```python
from build123d import *

# Parameters (mm, degrees)
EXTRUDE_1_DEPTH     = 6.6
SKETCH_2_W          = 4
SKETCH_2_H          = 1.1
CUT_EXTRUDE_1_DEPTH = 6.6
EXTRUDE_2_DEPTH     = 1
SKETCH_4_W          = 3.4
SKETCH_4_H          = 0.4
EXTRUDE_3_DEPTH     = 3.9
CHAMFER_1_SIZE      = 0.1
CHAMFER_1_SIZE2     = 0.173205081
SKETCH_5_W          = 8
SKETCH_5_H          = 1.5
SKETCH_5_W_2        = 2
SKETCH_5_H_2        = 1.9
CUT_EXTRUDE_2_DEPTH = 1.4
SKETCH_6_W          = 0.25
SKETCH_6_H          = 0.8
SKETCH_6_H_2        = 0.9
EXTRUDE_5_DEPTH     = 2.6
SKETCH_7_W          = 0.25
SKETCH_7_H          = 0.4
EXTRUDE_6_DEPTH     = 1.4
SKETCH_8_W          = 0.3
SKETCH_8_H          = 0.2
EXTRUDE_7_DEPTH     = 1.4
SKETCH_9_W          = 0.3
SKETCH_9_H          = 3.7
EXTRUDE_8_DEPTH     = 0.01
SKETCH_10_W         = 2.6
SKETCH_10_H         = 1.6
EXTRUDE_9_DEPTH     = 0.25
FILLET_1_R          = 0.1


with BuildPart() as part:
    # 草图1 → 凸台-拉伸1 (new body)
    with BuildSketch(Plane.XY):
        with BuildLine():
            Line((-3.35, 1.15), (3.35, 1.15))
            ThreePointArc((3.35, 1.15), (3.597487373, 1.047487373), (3.7, 0.8))
            Line((3.7, 0.8), (3.7, 0.1))
            ThreePointArc((3.7, 0.1), (3.675237691, -0.029307557), (3.604454603, -0.140318237))
            Line((3.604454603, -0.140318237), (2.754454603, -1.040318237))
            ThreePointArc((2.754454603, -1.040318237), (2.638543526, -1.121412027), (2.5, -1.15))
            Line((2.5, -1.15), (-2.5, -1.15))
            ThreePointArc((-2.5, -1.15), (-2.638543526, -1.121412027), (-2.754454603, -1.040318237))
            Line((-2.754454603, -1.040318237), (-3.604454603, -0.140318237))
            ThreePointArc((-3.604454603, -0.140318237), (-3.675237691, -0.029307557), (-3.7, 0.1))
            Line((-3.7, 0.1), (-3.7, 0.8))
            ThreePointArc((-3.7, 0.8), (-3.597487373, 1.047487373), (-3.35, 1.15))
        make_face()
        with BuildLine():
            Line((-3.35, 0.9), (3.35, 0.9))
            ThreePointArc((3.35, 0.9), (3.420710678, 0.870710678), (3.45, 0.8))
            Line((3.45, 0.8), (3.45, 0.1))
            ThreePointArc((3.45, 0.1), (3.442925055, 0.063054984), (3.422701315, 0.031337647))
            Line((3.422701315, 0.031337647), (2.572701315, -0.868662353))
            ThreePointArc((2.572701315, -0.868662353), (2.539583865, -0.891832008), (2.5, -0.9))
            Line((2.5, -0.9), (-2.5, -0.9))
            ThreePointArc((-2.5, -0.9), (-2.539583865, -0.891832008), (-2.572701315, -0.868662353))
            Line((-2.572701315, -0.868662353), (-3.422701315, 0.031337647))
            ThreePointArc((-3.422701315, 0.031337647), (-3.442925055, 0.063054984), (-3.45, 0.1))
            Line((-3.45, 0.1), (-3.45, 0.8))
            ThreePointArc((-3.45, 0.8), (-3.420710678, 0.870710678), (-3.35, 0.9))
        make_face(mode=Mode.SUBTRACT)
    extrude(amount=EXTRUDE_1_DEPTH)

    # 草图2 → 切除-拉伸1 (cut)
    with BuildSketch(Plane.XZ.offset(1.15)):
        with Locations((0, 0.55)):
            Rectangle(SKETCH_2_W, SKETCH_2_H)
    extrude(amount=-CUT_EXTRUDE_1_DEPTH, mode=Mode.SUBTRACT)

    # 草图3 → 凸台-拉伸2 (add)
    with BuildSketch(Plane(origin=(0, 0, 1.1), x_dir=(-1, 0, 0), z_dir=(0, 0, -1))):
        with BuildLine():
            Line((2.572701315, -0.868662353), (3.422701315, 0.031337647))
            ThreePointArc((3.422701315, 0.031337647), (3.442925055, 0.063054984), (3.45, 0.1))
            Line((3.45, 0.1), (3.45, 0.8))
            ThreePointArc((3.45, 0.8), (3.420710678, 0.870710678), (3.35, 0.9))
            Line((3.35, 0.9), (-3.35, 0.9))
            ThreePointArc((-3.35, 0.9), (-3.420710678, 0.870710678), (-3.45, 0.8))
            Line((-3.45, 0.8), (-3.45, 0.1))
            ThreePointArc((-3.45, 0.1), (-3.442925055, 0.063054984), (-3.422701315, 0.031337647))
            Line((-3.422701315, 0.031337647), (-2.572701315, -0.868662353))
            ThreePointArc((-2.572701315, -0.868662353), (-2.539583865, -0.891832008), (-2.5, -0.9))
            Line((-2.5, -0.9), (2.5, -0.9))
            ThreePointArc((2.5, -0.9), (2.539583865, -0.891832008), (2.572701315, -0.868662353))
        make_face()
    extrude(amount=-EXTRUDE_2_DEPTH)

    # 草图4 → 凸台-拉伸3 (add)
    with BuildSketch(Plane.XY.offset(2.1)):
        with Locations((0, 0.4)):
            Rectangle(SKETCH_4_W, SKETCH_4_H)
    extrude(amount=EXTRUDE_3_DEPTH)

    # 倒角1
    chamfer_1_edges = [part.edges().sort_by_distance(p)[0] for p in [
        (0, 0.2, 6),
    ]]
    chamfer_1_side = [part.faces().sort_by_distance(p)[0] for p in [
        (0, 0.4, 6),
    ]]
    chamfer(chamfer_1_edges, length=CHAMFER_1_SIZE, length2=CHAMFER_1_SIZE2, reference=chamfer_1_side[0])

    # 草图5 → 切除-拉伸2 (cut)
    with BuildSketch(Plane.XZ.offset(1.15)):
        with Locations((0, 0.35)):
            Rectangle(SKETCH_5_W, SKETCH_5_H)
        with Locations((3, 4.05)):
            Rectangle(SKETCH_5_W_2, SKETCH_5_H_2)
        with Locations((-3, 4.05)):
            Rectangle(SKETCH_5_W_2, SKETCH_5_H_2)
    extrude(amount=-CUT_EXTRUDE_2_DEPTH, mode=Mode.SUBTRACT)

    # 草图6 → 凸台-拉伸5 (add)
    with BuildSketch(Plane.XZ.offset(-0.25)):
        with Locations((3.575, 0.4)):
            Rectangle(SKETCH_6_W, SKETCH_6_H)
        with Locations((3.575, 3.85)):
            Rectangle(SKETCH_6_W, SKETCH_6_H_2)
        with Locations((-3.575, 3.85)):
            Rectangle(SKETCH_6_W, SKETCH_6_H_2)
        with Locations((-3.575, 0.4)):
            Rectangle(SKETCH_6_W, SKETCH_6_H)
    extrude(amount=EXTRUDE_5_DEPTH)

    # 草图7 → 凸台-拉伸6 (add)
    with BuildSketch(Plane.XZ.offset(-0.25)):
        with Locations((3.575, 4.5)):
            Rectangle(SKETCH_7_W, SKETCH_7_H)
        with Locations((-3.575, 4.5)):
            Rectangle(SKETCH_7_W, SKETCH_7_H)
    extrude(amount=EXTRUDE_6_DEPTH)

    # 草图8 → 凸台-拉伸7 (add)
    with BuildSketch(Plane(origin=(0, 0, 1.4), x_dir=(-1, 0, 0), z_dir=(0, 0, -1))):
        with Locations((-0.65, -1.2)):
            Rectangle(SKETCH_8_W, SKETCH_8_H)
        with Locations((0, -1.2)):
            Rectangle(SKETCH_8_W, SKETCH_8_H)
        with Locations((0.65, -1.2)):
            Rectangle(SKETCH_8_W, SKETCH_8_H)
        with Locations((1.3, -1.2)):
            Rectangle(SKETCH_8_W, SKETCH_8_H)
        with Locations((-1.3, -1.2)):
            Rectangle(SKETCH_8_W, SKETCH_8_H)
    extrude(amount=EXTRUDE_7_DEPTH)

    # 草图9 → 凸台-拉伸8 (add)
    with BuildSketch(Plane.XZ.offset(-0.2)):
        with Locations((-1.3, 3.95)):
            Rectangle(SKETCH_9_W, SKETCH_9_H)
        with Locations((-0.65, 3.95)):
            Rectangle(SKETCH_9_W, SKETCH_9_H)
        with Locations((0, 3.95)):
            Rectangle(SKETCH_9_W, SKETCH_9_H)
        with Locations((0.65, 3.95)):
            Rectangle(SKETCH_9_W, SKETCH_9_H)
        with Locations((1.3, 3.95)):
            Rectangle(SKETCH_9_W, SKETCH_9_H)
    extrude(amount=EXTRUDE_8_DEPTH)

    # 草图10 → 凸台-拉伸9 (add)
    with BuildSketch(Plane(origin=(0, 0, 1.1), x_dir=(-1, 0, 0), z_dir=(0, 0, -1))):
        with Locations((0, 0.35)):
            Rectangle(SKETCH_10_W, SKETCH_10_H)
    extrude(amount=EXTRUDE_9_DEPTH)

    # 圆角1
    fillet_1_edges = [part.edges().sort_by_distance(p)[0] for p in [
        (3.575, -2.35, 0),
        (3.575, -2.35, 0.8),
        (3.575, -2.35, 3.4),
        (3.575, -2.35, 4.3),
        (-3.575, -2.35, 4.3),
        (-3.575, -2.35, 3.4),
        (-3.575, -2.35, 0.8),
        (-3.575, -2.35, 0),
        (3.575, -1.15, 4.3),
        (3.575, -1.15, 4.7),
        (-3.575, -1.15, 4.7),
        (-3.575, -1.15, 4.3),
        (0, 1.15, 0.85),
    ]]
    fillet(fillet_1_edges, radius=FILLET_1_R)


solid = part.part
```
The listing builds one solid part. Answer for the finished solid, in the listing's coordinates (mm). A direction names the side the tool comes from. Coordinates: 2 decimals unless noted, no trailing zeros. Write each loop counter-clockwise with the first axis right and the second up, starting at its lowest first coordinate (ties: lowest second). Pieces come first, ordered by that corner, then holes. Notation, with made-up numbers: M -3.5,-18 L 34.5,-18 A25 ccw 34.5,-4 Z; hole C 77.25,88 d5. An arc over 180 degrees is marked long. Use a Markdown table: item, result. Add a question column.
1. Given P1, Ø1, axis at x = -0.5, y = 0, coming from the -Z side, flat-ended and moving along its own axis, determine where the tip first touches the part or whether it passes through.
2. Section C-C (x = -1) is taken. Give the vertices of the cut face in (y, z).
3. Section D-D (z = 1.5) is taken. Give the vertices of the cut face in (x, y), plus the area to 3 significant figures.
4. Section B-B (z = 2.75) is taken. Count the separate pieces of the cut face and the enclosed holes in it, plus the area to 3 significant figures.
5. Section A-A (y = -1.55) is taken. Give the vertices of the cut face in (x, z).
6. Which of the six approach directions +Z, -Z, +X, -X, +Y, -Y give full straight-line access (tool end or side, diameter ignored) to faces 1 (the flat face through (0.35, 0.2, 3.94)), 2 (the flat face through (-3.17, -0.6, 5.79)), 3 (the flat face through (3.45, -0.8, 0.4))?
7. Straight lines are drawn through the part: line 1 along Y through (x, z) = (1, 3.5); line 2 along X through (y, z) = (-0.95, 4.5); line 3 along X through (y, z) = (-2.05, 4). For each, find the intervals that lie inside material, in ascending order. Write a range as [from, to].
Data:
| question | item | result |
|---|---|---|
| 1 | P1 | stops at z = 0.85 |
| 2 | outline | M -1.15,1.1 L -0.45,1.1 L -0.45,0.85 L 1.05,0.85 A0.1 ccw 1.15,0.95 L 1.15,6.6 L 0.9,6.6 L 0.9,2.1 L 0.6,2.1 L 0.6,6 L 0.3,6 L 0.2,5.83 L 0.2,2.1 L -0.9,2.1 L -0.9,6.6 L -1.15,6.6 Z |
| 3 | outline | M -3.7,0.1 A0.35 ccw -3.6,-0.14 L -2.75,-1.04 A0.35 ccw -2.5,-1.15 L 2.5,-1.15 A0.35 ccw 2.75,-1.04 L 3.6,-0.14 A0.35 ccw 3.7,0.1 L 3.7,0.8 A0.35 ccw 3.35,1.15 L -3.35,1.15 A0.35 ccw -3.7,0.8 Z |
| 3 | area | 15.8 mm2 |
| 4 | separate pieces | 2 |
| 4 | enclosed holes | 1 |
| 4 | area | 5.62 mm2 |
| 5 | outline | M -3.7,0 L -3.45,0 L -3.45,0.8 L -3.7,0.8 Z; M -3.7,3.4 L -3.45,3.4 L -3.45,4.3 L -3.7,4.3 Z; M 3.45,0 L 3.7,0 L 3.7,0.8 L 3.45,0.8 Z; M 3.45,3.4 L 3.7,3.4 L 3.7,4.3 L 3.45,4.3 Z |
| 6 | face 1 | +Z |
| 6 | face 2 | +Z, -X, -Y |
| 6 | face 3 | -Z, -Y |
| 7 | line 1 | y = [-1.15, -0.9], [0.2, 0.6], [0.9, 1.15] |
| 7 | line 2 | x = [-3.7, -3.45], [-2, 2], [3.45, 3.7] |
| 7 | line 3 | x = [-3.7, -3.45], [3.45, 3.7] |
